Autodesk Inventor part; units mm, degrees
ref_plane "YZ Plane" through (0, 0, 0) normal (1, 0, 0) x (0, 1, 0)
ref_plane "XZ Plane" through (0, 0, 0) normal (0, 1, 0) x (-1, 0, 0)
ref_plane "XY Plane" through (0, 0, 0) normal (0, 0, 1) x (1, 0, 0)
sketch "Sketch1" plane through (0, 0, 0) normal (0, 0, 1) x (1, 0, 0)
  line L0 (-6.766, 0.5868) -> (-24.8151, 0.5868)
  line L1 (-24.8151, 0.5868) -> (-24.8151, -4.4132)
  line L2 (-24.8151, -4.4132) -> (-4.8151, -4.4132)
  line L3 (-4.8151, -4.4132) -> (-4.8151, -24.4132)
  line L4 (-4.8151, -24.4132) -> (0.1849, -24.4132)
  line L5 (0.1849, -24.4132) -> (0.1849, -6.3641)
  line L6 (-6.766, 0.5868) -> (15.3105, 22.6633)
  line L7 (22.2614, 15.7124) -> (0.1849, -6.3641)
  circle A0 centre (19.4349, 19.8368) radius 1.85
  arc A1 (22.2614, 15.7124) -> (15.3105, 22.6633) centre (19.4349, 19.8368) ccw
  dimension "d0" = 20
  dimension "d1" = 20
  dimension "d2" = 5
  dimension "d3" = 5
  dimension "d7" = 24.25
  dimension "d8" = 24.25
  dimension "d9" = 3.7
  dimension "d18" = 5
  dimension "d19" = 135
extrude "Extrusion1" add sketch "Sketch1" along normal blind 30
ref_plane "Work Plane1" through (0, 0, 24) normal (0, 0, 1) x (1, 0, 0)
sketch "Sketch3" plane through (0, 0, 24) normal (0, 0, 1) x (1, 0, 0)
  circle A0 centre (19.4349, 19.8368) radius 1.85
  circle A1 centre (19.4349, 19.8368) radius 12.5
  point P0 (0, 0)
  dimension "d13" = 25
extrude "Extrusion3" cut sketch "Sketch3" against normal blind 18
sketch "Sketch5" plane through (0, 0, 0) normal (0, 0, -1) x (-1, 0, 0)
  circle A0 centre (-19.4349, 19.8368) radius 1.85
  line L0 (24.8151, -4.4132) -> (24.8151, 0.5868)
  line L1 (24.8151, 0.5868) -> (6.766, 0.5868)
  line L2 (6.766, 0.5868) -> (-15.3105, 22.6633)
  arc A1 (-15.3105, 22.6633) -> (-22.2614, 15.7124) centre (-19.4349, 19.8368) ccw
  line L3 (-22.2614, 15.7124) -> (-0.1849, -6.3641)
  line L4 (-0.1849, -6.3641) -> (-0.1849, -24.4132)
  line L5 (-0.1849, -24.4132) -> (4.8151, -24.4132)
  line L6 (4.8151, -24.4132) -> (4.8151, -4.4132)
  line L7 (4.8151, -4.4132) -> (24.8151, -4.4132)
  line L8 (-0.1849, -6.3641) -> (6.766, 0.5868)
  point P0 (0, 0)
extrude "Extrusion5" add sketch "Sketch5" along normal blind 25 contours L7 L6 L5 L4 L8 L1 L0
sketch "Sketch8" plane through (-4.8151, -24.4132, -25) normal (-1, 0, 0) x (0, 0, 1)
  circle A0 centre (10, 10) radius 2.25
  line L0 (55, 0) -> (0, 0)
  line L1 (0, 0) -> (0, 20)
  circle A1 centre (25, 10) radius 2.25
  point P0 (25, 24.4132)
  dimension "d40" = 4.5
  dimension "d41" = 10
  dimension "d42" = 10
  dimension "d43" = 4.5
  dimension "d44" = 10
  dimension "d45" = 15
sketch "Sketch9" plane through (-24.8151, 0.5868, 30) normal (0, 1, 0) x (1, 0, 0)
  circle A0 centre (10, 45) radius 2.25
  circle A1 centre (10, 30) radius 2.25
  line L0 (0, 55) -> (18.0491, 55)
  line L1 (0, 0) -> (0, 55)
  point P0 (24.8151, 30)
  dimension "d46" = 10
  dimension "d47" = 10
  dimension "d48" = 10
  dimension "d49" = 15
  dimension "d50" = 4.5
  dimension "d51" = 4.5
extrude "Extrusion8" cut sketch "Sketch9" against normal mid plane 20
extrude "Extrusion9" cut sketch "Sketch8" against normal blind 20
sketch "Sketch10" plane through (0, 0, 30) normal (0, 0, 1) x (1, 0, 0)
  line L0 (-3.9108, 3.9108) -> (4.5333, -4.5333)
  line L1 (4.5333, -4.5333) -> (4.5333, -31.01)
  line L2 (4.5333, -31.01) -> (-28.169, -31.01)
  line L3 (-28.169, -31.01) -> (-28.169, 3.9108)
  line L4 (-28.169, 3.9108) -> (-3.9108, 3.9108)
  point P0 (0, 0)
  dimension "d56" = 135
  dimension "d57" = 0
extrude "Extrusion10" cut sketch "Sketch10" against normal blind 15
equation "\"d8\" = d7"
equation "\"d43\" = d40"
equation "\"d44\" = d41"
equation "\"RodDiameter\" = 8"
equation "\"VerticalBearingOD\" = 16"
equation "\"PrintingClearance\" = 0.2"
equation "\"TubeID\" = 18"
properties part number "PulleyHolderXY"
Work out the finished part from the listing and answer in its coordinate system (mm). A direction names the side the tool comes from. Round coordinates to 2 decimals unless told otherwise and drop trailing zeros. Loops run counter-clockwise (first coordinate to the right, second up) from the corner with the lowest first, then second, coordinate; pieces in that order, holes last. Notation, with made-up numbers: (78, -10.5) -> (93, -10.5) arc R17 cw to (93, 8.5) -> close; hole circle Ø10 at (2, 32). An arc over 180 degrees is marked (long way). Write each question's results on one line, items separated by ' | '. Start each with the question number.
1. For a pull along Y with two mould halves and no side action, classify faces 1 (the face through (-2.35, -16.61, -0.49)), 2 (the face through (-4, -7, -25)), 3 (the face through (-3.24, -2.94, -12.32)), 4 (the face through (19.2, 18, 3)) as +Y half, -Y half, draft (parallel to the pull), parting line (faces both ways), or undercut.
2. Given pin 1 Ø14.5 at (y, z) = (-14.5, -1) entering from +X; pin 2 Ø16 at (y, z) = (-18, -7) entering from -X; pin 3 Ø5 at (x, z) = (-14.82, -15) entering from -Y; pin 4 Ø10 at (y, z) = (17, 4.5) entering from +X, each flat-ended and moving along its own axis, determine where each tip first touches the part or whether it passes through.
3. A tool of negligible diameter and unlimited length cuts with its end or side. For faces 5 (the face through (-4.815, -15, -5)), 6 (the face through (10.546, 11.048, 15.126)), 7 (the face through (-8, -4, 15)), from which of +Z, -Z, +X, -X, +Y, -Y can it reach the whole face along a straight path? Write none if from no direction.
4. Find the intervals of material crossed by probe 1 along Z at (x, y) = (13.5, 18.5); probe 2 along X at (y, z) = (-17, 8); probe 3 along Y at (x, z) = (-11, -15), in increasing order. Write a range as from..to.
5. Section C-C (x = -6) is taken. Determine the outline of the cut face in (y, z), plus the area to 3 significant figures.
6. Section A-A (z = -15) is taken. Determine the outline of the cut face in (x, y).
7. Section B-B (y = -13) is taken. Determine the outline of the cut face in (x, z).
Evaluation:
1) face 1: undercut | face 2: draft | face 3: +Y half | face 4: undercut
2) pin 1: stops at x = 0.18 | pin 2: stops at x = -4.82 | pin 3: stops at y = -4.41 | pin 4: stops at x = 24.43
3) face 5: +Z, -Z, -X, -Y | face 6: +X, +Y | face 7: +Z, -X, -Y
4) probe 1: z = 0..6, 24..30 | probe 2: x = -4.82..0.18 | probe 3: y = -4.41..0.59
5) outline: (-4.41, -25) -> (-0.18, -25) -> (-0.18, 0) -> (1.35, 0) -> (1.35, 15) -> (-4.41, 15) -> close | area: 192 mm2
6) outline: (-24.82, -4.41) -> (-17.07, -4.41) -> (-17.07, 0.59) -> (-24.82, 0.59) -> close; (-12.57, -4.41) -> (-4.82, -4.41) -> (-4.82, -12.16) -> (0.18, -12.16) -> (0.18, -6.36) -> (-6.77, 0.59) -> (-12.57, 0.59) -> close; (-4.82, -24.41) -> (0.18, -24.41) -> (0.18, -16.66) -> (-4.82, -16.66) -> close
7) outline: (-4.82, -25) -> (0.18, -25) -> (0.18, -16.75) -> (-4.82, -16.75) -> close; (-4.82, -13.25) -> (0.18, -13.25) -> (0.18, -1.75) -> (-4.82, -1.75) -> close; (-4.82, 1.75) -> (0.18, 1.75) -> (0.18, 15) -> (-4.82, 15) -> close
